Source: CAD feature listing. Evaluate the final solid. Frame: model axes, mm. Face numbers are marked on the shaded views. A direction names the side the tool comes from. Coordinates: 2 decimals unless noted, no trailing zeros. Order: outer loops, then holes, each group sorted by start corner. A loop starts at its lowest first (then second) coordinate and runs counter-clockwise, first axis right, second up. Notation, with made-up numbers: (70, 30.25) - (80, 30.25) arc R11 cw to (80, 39.25) - close; hole circle Ø9 at (66, -36). An arc over 180 degrees is marked (long way). One line per question, with ' | ' between items.
Autodesk Inventor part; units mm, degrees
ref_plane "YZ Plane" through (0, 0, 0) normal (1, 0, 0) x (0, 1, 0)
ref_plane "XZ Plane" through (0, 0, 0) normal (0, 1, 0) x (-1, 0, 0)
ref_plane "XY Plane" through (0, 0, 0) normal (0, 0, 1) x (1, 0, 0)
sketch "Sketch1" plane through (0, 0, 0) normal (0, 1, 0) x (-1, 0, 0)
  circle A0 centre (0, 0) radius 80
  circle A1 centre (0, 0) radius 7.5
  dimension "d0" = 160
  dimension "d1" = 15
extrude "Extrusion1" add sketch "Sketch1" along normal blind 10
sketch "Sketch2" plane through (0, 10, 0) normal (0, 1, 0) x (1, 0, 0)
  circle A0 centre (0, 0) radius 7.5
  line L0 (0, -7.5) -> (-40, -7.5)
  line L1 (-40, -7.5) -> (-40, -27.5)
  line L2 (-40, -27.5) -> (0, -27.5)
  line L3 (0, -27.5) -> (0, -7.5)
  line L4 (0, -27.5) -> (40, -27.5)
  line L5 (40, -27.5) -> (40, -7.5)
  line L6 (40, -7.5) -> (0, -7.5)
  line L7 (0, -7.5) -> (0, -27.5)
  dimension "d4" = 40
  dimension "d5" = 20
  dimension "d6" = 40
extrude "Extrusion2" add sketch "Sketch2" along normal blind 150 contours L6 L5 L4 L3 | L3 L2 L1 L0
sketch "Sketch3" plane through (-40, 10, 27.5) normal (0, 0, 1) x (1, 0, 0)
  circle A0 centre (40, 75) radius 25
  line L0 (0, 150) -> (80, 150)
  line L1 (80, 0) -> (80, 150)
  line L2 (0, 150) -> (80, 150)
  line L3 (80, 150) -> (80, 105)
  line L4 (80, 105) -> (0, 105)
  line L5 (0, 105) -> (0, 150)
  line L6 (0, 0) -> (0, 150)
  arc A1 (40, 105) -> (0, 75) centre (38.735, 65.02) ccw
  arc A2 (80, 75) -> (40, 105) centre (41.265, 65.02) ccw
  point P0 (40, -10)
  dimension "d9" = 50
  dimension "d10" = 45
  dimension "d11" = 40
  dimension "d12" = 40
extrude "Extrusion3" cut sketch "Sketch3" against normal blind 21.45 contours A0 | L0 L1 L4 A2 A1 L5 | L4 A1 L6 | L1 A2 L4
sketch "Sketch4" plane through (-40, 10, 27.5) normal (0, 0, 1) x (1, 0, 0)
  point P0 (40, -10)
properties part number "Base Top"
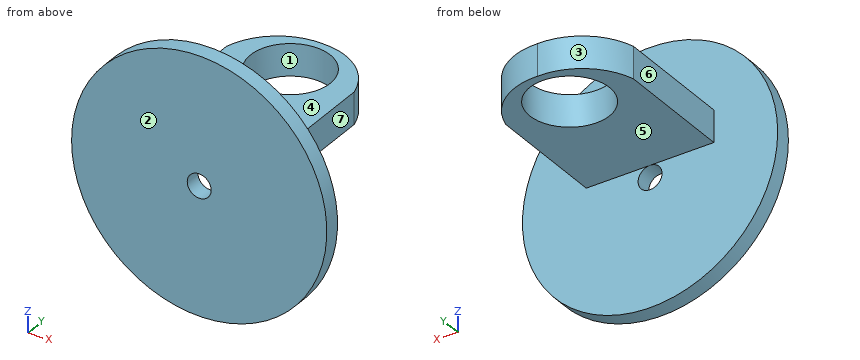
(1) Cut plane C-C (z = 22). Return the cut outline in (x, y) (3 decimals), and give its area (3 significant figures).
Taken from the geometry:
outline: (-76.916, 0) - (76.916, 0) - (76.916, 10) - (40, 10) - (40, 85) arc R40 ccw to (0, 115) arc R40 ccw to (-40, 85) - (-40, 10) - (-76.916, 10) - close; hole circle Ø50 at (0, 85) | area: 7,370 mm²
(2) Material intervals for L1, parallel to Y at x = 0, z = 18.75; L2, parallel to Z at x = 0, y = 6; L3, parallel to Y at x = 7, z = -12.5, sorted ascending. Write a range as from..to.
Taken from the geometry:
L1: y = 0..60, 110..115 | L2: z = -80..-7.5, 7.5..80 | L3: y = 0..10
(3) Pull-direction query (Y, two-part tool) for the marked faces 1, 2 and 3; classes: pulls with the +Y half, pulls with the -Y half, needs draft (parallel to the pull), parting line crosses it, or undercut.
Taken from the geometry:
face 1: undercut | face 2: pulls with the -Y half | face 3: pulls with the +Y half
(4) Pin query (flat end, axial travel): P1, Ø24, axis at x = -12.5, y = 62, coming from the +Z side; P2, Ø5, axis at x = 36, z = 1.5, coming from the +Y side; P3, Ø9, axis at x = 0, z = 0, coming from the +Y side; P4, Ø6, axis at y = 37.5, z = 19, coming from the +X side. Return the tip coordinate at first contact, or that it passes through.
Taken from the geometry:
P1: stops at z = 27.5 | P2: stops at y = 10 | P3: passes through | P4: stops at x = 40
(5) Cut plane A-A (y = 65). Return the cut outline in (x, z), and give its area (3 significant figures).
Taken from the geometry:
outline: (-40, 7.5) - (-15, 7.5) - (-15, 27.5) - (-40, 27.5) - close; (15, 7.5) - (40, 7.5) - (40, 27.5) - (15, 27.5) - close | area: 1,000 mm²
(6) Cut plane B-B (z = 0). Return the cut outline in (x, y).
Taken from the geometry:
outline: (-80, 0) - (-7.5, 0) - (-7.5, 10) - (-80, 10) - close; (7.5, 0) - (80, 0) - (80, 10) - (7.5, 10) - close
(7) Set-up query: the marked faces 4, 5, 6 and 7. Return all of +Z, -Z, +X, -X, +Y, -Y with unobstructed straight access to the full face (end or side cutting, diameter ignored); none if empty.
Taken from the geometry:
face 4: +Z, +X, -X, +Y | face 5: -Z, +X, -X, +Y | face 6: +Z, -Z, -X, +Y | face 7: +Z, -Z, +X, +Y
(8) Cut plane D-D (y = 7). Return the cut outline in (x, z).
Taken from the geometry:
outline: circle Ø160 at (0, 0); hole circle Ø15 at (0, 0)
